from build123d import *
from OCP.BRepFilletAPI import BRepFilletAPI_MakeChamfer

# Parameters (mm, degrees)
SKETCH1_R           = 5.75
BOSS_EXTRUDE1_DEPTH = 3
BOSS_EXTRUDE2_DEPTH = 0.25
CIRPATTERN2_COUNT   = 2
SKETCH5_R           = 2.5
CUT_EXTRUDE2_DEPTH  = 65.81337733
CHAMFER1_SIZE       = 1
CHAMFER1_SIZE2      = 1.191753593
CIRPATTERN1_COUNT   = 2


with BuildPart() as part:
    # Sketch1 → Boss-Extrude1 (new, symmetric)
    with BuildSketch(Plane(origin=(0, 0, 0), x_dir=(1, 0, 0), z_dir=(0, 1, 0))):
        with Locations(Location((0, 0, 0), (0, 0, 270))):
            Circle(SKETCH1_R)
    extrude(amount=BOSS_EXTRUDE1_DEPTH, both=True)

    # Sketch3 → Boss-Extrude2 (add, symmetric)
    with BuildSketch(Plane(origin=(0, 0, 0), x_dir=(0.9743700647852351, -0.22495105434386545, 0), z_dir=(-0.22495105434386545, -0.9743700647852351, 0))):
        with BuildLine():
            Line((-4.217884967, 2.801368956), (-11.756994241, 6.527912594))
            Line((-11.756994241, 6.527912594), (-11.756994241, 60.5))
            ThreePointArc((-11.756994241, 60.5), (-10.878314584, 62.621320344), (-8.756994241, 63.5))
            Line((-8.756994241, 63.5), (-6.892338734, 63.5))
            ThreePointArc((-6.892338734, 63.5), (-3.698351895, 62.346875105), (-1.977591351, 59.419379228))
            add(Edge.make_bspline(
                [(-1.977591351, 59.419379228), (8.598166734, 31.505186927), (4.658441713, 1.76136177)],
                knots=[0, 0, 0, 1, 1, 1], degree=2))
            add(Edge.make_bspline(
                [(-4.217884967, 2.801368956), (1.070543738, 9.225844279), (4.658441713, 1.76136177)],
                knots=[0, 0, 0, 1, 1, 1], degree=2))
        make_face()
    boss_extrude2 = extrude(amount=BOSS_EXTRUDE2_DEPTH, both=True)

    # CirPattern2: Boss-Extrude2 ×2 about axis
    cirpattern2_axis = Axis((0, 3, 0), (0, -1, 0))
    for i in range(1, CIRPATTERN2_COUNT):
        add(boss_extrude2.rotate(cirpattern2_axis, i * 360 / CIRPATTERN2_COUNT))

    # Sketch5 → Cut-Extrude2 (cut, through all)
    with BuildSketch(Plane.XZ.offset(3)):
        with Locations(Location((0, 0, 0), (0, 0, 270))):
            Circle(SKETCH5_R)
    extrude(amount=-CUT_EXTRUDE2_DEPTH, mode=Mode.SUBTRACT)

    # Chamfer1: one chamfer whose edges measure the first distance from different faces: ONE call of the kernel's chamfer builder (chamfer() names one face for all edges)
    chamfer1_edges_1 = [part.edges().sort_by_distance(p)[0] for p in [
        (0, 3, 2.5),
    ]]
    chamfer1_side_1 = [part.faces().sort_by_distance(p)[0] for p in [
        (0, 0, 2.5),
    ]]
    chamfer1_edges_2 = [part.edges().sort_by_distance(p)[0] for p in [
        (0, -3, 2.5),
    ]]
    chamfer1_side_2 = [part.faces().sort_by_distance(p)[0] for p in [
        (0, -3, -5.58736544),
    ]]
    chamfer1 = BRepFilletAPI_MakeChamfer(part.part.solid().wrapped)
    for e in chamfer1_edges_1:
        chamfer1.Add(CHAMFER1_SIZE, CHAMFER1_SIZE2, e.wrapped, chamfer1_side_1[0].wrapped)  # the first distance lies on this face
    for e in chamfer1_edges_2:
        chamfer1.Add(CHAMFER1_SIZE, CHAMFER1_SIZE2, e.wrapped, chamfer1_side_2[0].wrapped)  # the first distance lies on this face
    add(Compound.cast(chamfer1.Shape()), mode=Mode.REPLACE)

    # CirPattern1: Boss-Extrude2 ×2 about axis
    cirpattern1_axis = Axis((0, 3, 0), (0, -1, 0))
    for i in range(1, CIRPATTERN1_COUNT):
        add(boss_extrude2.rotate(cirpattern1_axis, i * 360 / CIRPATTERN1_COUNT))


solid = part.part
Read the model definition and answer for the solid it produces. Units are mm, in the model's axes. A direction names the side the tool comes from. Coordinates: 2 decimals unless noted, no trailing zeros. Loops run counter-clockwise (first coordinate to the right, second up) from the corner with the lowest first, then second, coordinate; pieces in that order, holes last. Notation, with made-up numbers: (32, 88.5) -> (88, 88.5) arc R9 ccw to (88, 102.5) -> close; hole circle Ø8 at (74, 40.25). An arc over 180 degrees is marked (long way). Answer in a Markdown table with one row per item.
Item 1: Each of these flat-tipped pins is pushed along its axis until it touches: P1, Ø3, axis at x = -8, y = -2, coming from the +Z side; P2, Ø6.5, axis at x = 0, z = 0, coming from the +Y side; P3, Ø3, axis at x = -1, y = 0, coming from the +Z side; P4, Ø1.5, axis at x = -3.5, z = -7.5, coming from the +Y side. Where does it stop, or does it pass through?
Returned:
| item | result |
|---|---|
| P1 | passes through |
| P2 | stops at y = 2.63 |
| P3 | stops at z = 60.84 |
| P4 | stops at y = -0.38 |
Item 2: For faces 1 (the flat face through (0, -3, 4)), 2 (the cylindrical face through (1.727, 0.042, 5.484)), determine the directions among +Z, -Z, +X, -X, +Y, -Y from which every point of the face is accessible in a straight line to the end or side of a thin tool.
Returned:
| item | result |
|---|---|
| face 1 | +Z, -Z, +X, -X, -Y |
| face 2 | none |
Item 3: A cutting plane is placed at A-A on z = 0. Determine the outline of the cut face in (x, y).
Returned:
| item | result |
|---|---|
| outline | (-5.75, -3) -> (-3.5, -3) -> (-2.5, -1.81) -> (-2.5, 2) -> (-3.69, 3) -> (-5.75, 3) -> close; (2.5, -1.81) -> (3.5, -3) -> (5.75, -3) -> (5.75, 3) -> (3.69, 3) -> (2.5, 2) -> close |
Item 4: Straight lines are drawn through the part: line 1 along X through (y, z) = (-0.2, 0); line 2 along Y through (x, z) = (9.75, -53.5); line 3 along Z through (x, y) = (-0.5, 1.5). For each, find the intervals that lie inside material, in ascending order. Write a range as [from, to].
Returned:
| item | result |
|---|---|
| line 1 | x = [-5.75, -2.5], [2.5, 5.75] |
| line 2 | y = [1.99, 2.51] |
| line 3 | z = [-5.73, -2.45], [2.45, 5.73] |
